from build123d import *

# Parameters (mm, degrees)
SKETCH1_W           = 30
SKETCH1_H           = 80
BOSS_EXTRUDE1_DEPTH = 10
SKETCH2_R           = 15
BOSS_EXTRUDE2_DEPTH = 20
SKETCH3_R           = 10
CUT_EXTRUDE1_DEPTH  = 5


with BuildPart() as part:
    # Sketch1 → Boss-Extrude1 (new body)
    with BuildSketch(Plane(origin=(0, 0, 0), x_dir=(1, 0, 0), z_dir=(0, 1, 0))):
        Rectangle(SKETCH1_W, SKETCH1_H)
    extrude(amount=BOSS_EXTRUDE1_DEPTH)

    # Sketch2 → Boss-Extrude2 (add)
    with BuildSketch(Plane(origin=(0, 10, 0), x_dir=(1, 0, 0), z_dir=(0, 1, 0))):
        with Locations((0, 25)):
            Circle(SKETCH2_R)
    extrude(amount=BOSS_EXTRUDE2_DEPTH)

    # Sketch3 → Cut-Extrude1 (cut)
    with BuildSketch(Plane(origin=(0, 10, 0), x_dir=(1, 0, 0), z_dir=(0, 1, 0))):
        with Locations((0, -25)):
            Circle(SKETCH3_R)
    extrude(amount=-CUT_EXTRUDE1_DEPTH, mode=Mode.SUBTRACT)


solid = part.part
Model file for the job. Use its own axes, mm. A direction names the side the tool comes from. Give positions to 0.01 mm unless a question says otherwise; leave off trailing zeros. Loops run counter-clockwise (first coordinate to the right, second up) from the corner with the lowest first, then second, coordinate; pieces in that order, holes last. Notation, with made-up numbers: (-20, 59.25) -> (10, 59.25) arc R10 cw to (10, 73.25) -> close; hole circle Ø2 at (1.25, 10). An arc over 180 degrees is marked (long way). Use a Markdown table: item, result. Add a question column.
(1) Tool access for faces 5 (the cylindrical face through (-3.252, 19.86, -10.357)), 6 (the flat face through (-12, 10, -36)), 7 (the flat face through (11, 10, -37)), 8 (the flat face through (0, 30, -25)): list every direction of +Z, -Z, +X, -X, +Y, -Y with a clear straight run to the whole face (end or side of a thin tool).
(2) Slice it at A-A on z = 25. List the corners of the cut face in (x, y).
(3) Mould opens along X. For faces 1 (the cylindrical face through (5.38, 7.54, 16.57)), 2 (the flat face through (0, 5, 25)), 3 (the flat face through (-15, 5, 1)), 4 (the flat face through (0, 5, -40)) say: +X half, -X half, draft (parallel to the pull), parting line (faces both ways), or undercut.
(4) Slice it at C-C on y = 17. List the corners of the cut face in (x, z).
(5) Wall check: line 1 along X through (y, z) = (8.9, 25); line 2 along Z through (x, y) = (0, 7); line 3 along Y through (x, z) = (-2, 20). Give the ranges that are in metal, low to high.
(6) Drop flat-ended pins along their axis: pin 1 Ø5 at (x, y) = (-8, 13) entering from -Z; pin 2 Ø16 at (x, z) = (0, 25) entering from -Y; pin 3 Ø10 at (x, z) = (-2.5, 4.5) entering from +Y. Give the stop position or say it passes through.
(7) Slice it at B-B on x = 3.5. List the corners of the cut face in (y, z), and give its area (3 significant figures).
(8) Slice it at D-D on z = -31.5. List the corners of the cut face in (x, y), and give its area (3 significant figures).
Filled sheet:
| question | item | result |
|---|---|---|
| 1 | face 5 | +Y |
| 1 | face 6 | -Z, -X, +Y |
| 1 | face 7 | -Z, +X, +Y |
| 1 | face 8 | +Z, -Z, +X, -X, +Y |
| 2 | outline | (-15, 0) -> (15, 0) -> (15, 10) -> (10, 10) -> (10, 5) -> (-10, 5) -> (-10, 10) -> (-15, 10) -> close |
| 3 | face 1 | undercut |
| 3 | face 2 | undercut |
| 3 | face 3 | -X half |
| 3 | face 4 | draft |
| 4 | outline | circle Ø30 at (0, -25) |
| 5 | line 1 | -15 to -10, 10 to 15 |
| 5 | line 2 | -40 to 15, 35 to 40 |
| 5 | line 3 | 0 to 5 |
| 6 | pin 1 | z = -38.96 |
| 6 | pin 2 | y = 0 |
| 6 | pin 3 | y = 10 |
| 7 | outline | (0, -40) -> (10, -40) -> (10, -39.59) -> (30, -39.59) -> (30, -10.41) -> (10, -10.41) -> (10, 15.63) -> (5, 15.63) -> (5, 34.37) -> (10, 34.37) -> (10, 40) -> (0, 40) -> close |
| 7 | area | 1,290 mm2 |
| 8 | outline | (-15, 0) -> (15, 0) -> (15, 10) -> (13.52, 10) -> (13.52, 30) -> (-13.52, 30) -> (-13.52, 10) -> (-15, 10) -> close |
| 8 | area | 841 mm2 |
